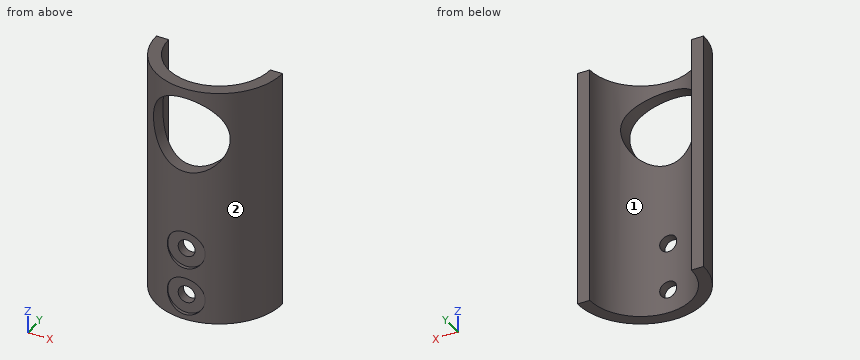
```python
from build123d import *

# Parameters (mm, degrees)
BOSS_EXTRUDE1_DEPTH     = 63.5
CUT_EXTRUDE1_REACH      = 69.75
CUT_EXTRUDE1_END_RADIUS = 16.7005
SKETCH2_R               = 10.16
CUT_EXTRUDE2_REACH      = 69.75
CUT_EXTRUDE2_END_RADIUS = 16.7005
SKETCH5_R               = 2.25
SKETCH8_R               = 5
CUT_EXTRUDE4_DEPTH      = 2.032


with BuildPart() as part:
    # Sketch1 → Boss-Extrude1 (new body)
    with BuildSketch(Plane.XY):
        with BuildLine():
            ThreePointArc((13.462, 0), (0, -13.462), (-13.462, 0))
            Line((-13.462, 0), (-16.7005, 0))
            ThreePointArc((-16.7005, 0), (0, -16.7005), (16.7005, 0))
            Line((16.7005, 0), (13.462, 0))
        make_face()
    extrude(amount=BOSS_EXTRUDE1_DEPTH)

    # Cut-Extrude1: up to this cylinder (the profile starts inside it)
    cut_extrude1_end = Plane(origin=(0, 0, 50.8), z_dir=(0, 0, -1)) * Cylinder(CUT_EXTRUDE1_END_RADIUS, 173.901, mode=Mode.PRIVATE)
    # Sketch2 → Cut-Extrude1 (cut, up to the surface)
    with BuildSketch(Plane(origin=(0, 0, 0), x_dir=(1, 0, 0), z_dir=(0, 1, 0)), mode=Mode.PRIVATE) as cut_extrude1_sk1:
        with Locations(Location((0, -50.8, 0), (0, 0, 270))):
            Circle(SKETCH2_R)
    cut_extrude1_tool1 = extrude(cut_extrude1_sk1.sketch, amount=-CUT_EXTRUDE1_REACH, mode=Mode.PRIVATE) & cut_extrude1_end
    add(cut_extrude1_tool1.solids().sort_by_distance((0, 0, 50.8))[0], mode=Mode.SUBTRACT)

    # Cut-Extrude2: up to this cylinder (the profile starts inside it)
    cut_extrude2_end = Plane(origin=(0, 0, 12.7), z_dir=(0, 0, -1)) * Cylinder(CUT_EXTRUDE2_END_RADIUS, 186.601, mode=Mode.PRIVATE)
    # Sketch5 → Cut-Extrude2 (cut, up to the surface)
    with BuildSketch(Plane(origin=(0, 0, 0), x_dir=(1, 0, 0), z_dir=(0, 1, 0)), mode=Mode.PRIVATE) as cut_extrude2_sk1:
        with Locations(Location((0, -6.35, 0), (0, 0, 270))):
            Circle(SKETCH5_R)
    cut_extrude2_tool1 = extrude(cut_extrude2_sk1.sketch, amount=-CUT_EXTRUDE2_REACH, mode=Mode.PRIVATE) & cut_extrude2_end
    add(cut_extrude2_tool1.solids().sort_by_distance((0, 0, 6.35))[0], mode=Mode.SUBTRACT)
    # Sketch5 → Cut-Extrude2 (cut, up to the surface)
    with BuildSketch(Plane(origin=(0, 0, 0), x_dir=(1, 0, 0), z_dir=(0, 1, 0)), mode=Mode.PRIVATE) as cut_extrude2_sk2:
        with Locations(Location((0, -19.05, 0), (0, 0, 270))):
            Circle(SKETCH5_R)
    cut_extrude2_tool2 = extrude(cut_extrude2_sk2.sketch, amount=-CUT_EXTRUDE2_REACH, mode=Mode.PRIVATE) & cut_extrude2_end
    add(cut_extrude2_tool2.solids().sort_by_distance((0, 0, 19.05))[0], mode=Mode.SUBTRACT)

    # Sketch8 → Cut-Extrude4 (cut)
    with BuildSketch(Plane(origin=(0, -17.78, 0), x_dir=(1, 0, 0), z_dir=(0, 1, 0))):
        with Locations(Location((0, -6.35, 0), (0, 0, 90))):
            Circle(SKETCH8_R)
        with Locations(Location((0, -19.05, 0), (0, 0, 90))):
            Circle(SKETCH8_R)
    extrude(amount=CUT_EXTRUDE4_DEPTH, mode=Mode.SUBTRACT)


solid = part.part
```
Model file for the job. Use its own axes, mm. Face numbers are marked on the shaded views. Round coordinates to 2 decimals unless told otherwise and drop trailing zeros. Loops run counter-clockwise (first coordinate to the right, second up) from the corner with the lowest first, then second, coordinate; pieces in that order, holes last. Notation, with made-up numbers: M -10,-11 L -4,-11 A26 ccw -4,3 Z; hole C -37,-16 d11. An arc over 180 degrees is marked long. Put each result on its own line as item: value. Start each with the question number.
Item 1: Cut at B-B (z = 47). List the corners of the cut face in (x, y).
Item 2: Cut at C-C (y = -12.25). List the corners of the cut face in (x, z), then the cut area to 3 significant figures.
Item 3: Cut at A-A (x = -9). List the corners of the cut face in (y, z), then the cut area to 3 significant figures.
Item 4: Drill centre lines: line 1 along Z through (x, y) = (0, -14.85); line 2 along X through (y, z) = (-0.5, 57); line 3 along X through (y, z) = (-12.5, 50.8). Where is each one in solid material? Low to high.
Item 5: Cut at D-D (z = 19.05). List the corners of the cut face in (x, y), then the cut area to 3 significant figures.
Item 6: Mould opens along X. For the marked faces 1 and 2 say: released by +X, released by -X, zero draft, split by the parting line, or undercut.
Item 7: Drop flat-ended pins along their axis: P1, Ø1, axis at y = -11.5, z = 36, coming from the +X side; P2, Ø5, axis at x = -11.5, y = -11, coming from the -Z side; P3, Ø8, axis at x = 0, z = 6.35, coming from the +Y side; P4, Ø5, axis at x = -10, z = 15, coming from the -Y side. Give the stop position or say it passes through.
Answer block:
1. outline: M -16.7,0 A16.7 ccw -9.42,-13.79 L -9.42,-9.61 A13.46 cw -13.46,0 Z; M 9.42,-13.79 A16.7 ccw 16.7,0 L 13.46,0 A13.46 cw 9.42,-9.61 Z
2. outline: M -11.35,0 L -5.58,0 L -5.58,42.31 A10.16 cw -5.58,59.29 L -5.58,63.5 L -11.35,63.5 Z; M 5.58,0 L 11.35,0 L 11.35,63.5 L 5.58,63.5 L 5.58,59.29 A10.16 cw 5.58,42.31 Z
2. area: 623 mm2
3. outline: M -14.07,0 L -10.01,0 L -10.01,46.09 L -14.07,46.09 Z; M -14.07,55.51 L -10.01,55.51 L -10.01,63.5 L -14.07,63.5 Z
3. area: 219 mm2
4. line 1: 0 to 4.1, 8.6 to 16.8, 21.3 to 40.64, 60.96 to 63.5
4. line 2: -16.69 to -13.45, 13.45 to 16.69
4. line 3: -11.08 to -10.16, 10.16 to 11.08
5. outline: M -16.7,0 A16.7 ccw -5,-15.93 L -5,-15.75 L -2.25,-15.75 L -2.25,-13.27 A13.46 cw -13.46,0 Z; M 2.25,-15.75 L 5,-15.75 L 5,-15.93 A16.7 ccw 16.7,0 L 13.46,0 A13.46 cw 2.25,-13.27 Z
5. area: 136 mm2
6. face 1: undercut
6. face 2: split by the parting line
7. P1: x = 12.57
7. P2: z = 0
7. P3: y = -12.85
7. P4: y = -14.92
